Can you work these out from the model? Positions are in its coordinate system, mm. Face numbers are marked on the shaded views. A direction names the side the tool comes from. Coordinates: 2 decimals unless noted, no trailing zeros. Loops run counter-clockwise (first coordinate to the right, second up) from the corner with the lowest first, then second, coordinate; pieces in that order, holes last.
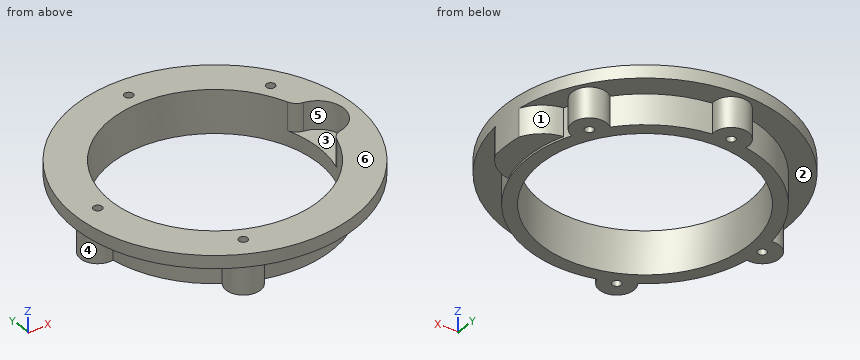
```python
from build123d import *

# Parameters (mm, degrees)
SKETCH1_R                = 32.5
SKETCH1_R_2              = 24.1
SKETCH1_R_3              = 1
RING_BODY_DEPTH          = 10
SKETCH2_R                = 6
NUB_CUT_DEPTH            = 6.5
NUB_CUT_FILLETS_3MM_R    = 3
WEIGHT_REDUCTION_DEPTH   = 7
WEIGHT_REDUCTION_2_DEPTH = 0.5


# Read off the part's stored shape, not the designer's step: Weight reduction
with BuildPart() as part:
    # Sketch1 → Ring body (new body)
    with BuildSketch(Plane.XY):
        Circle(SKETCH1_R)
        Circle(SKETCH1_R_2, mode=Mode.SUBTRACT)
        with Locations((0, 27.5)):
            Circle(SKETCH1_R_3, mode=Mode.SUBTRACT)
        with Locations((23.5226917, 14.245454545)):
            Circle(SKETCH1_R_3, mode=Mode.SUBTRACT)
        with Locations((-27.5, 0)):
            Circle(SKETCH1_R_3, mode=Mode.SUBTRACT)
        with Locations((-11.677272727, -24.897616385)):
            Circle(SKETCH1_R_3, mode=Mode.SUBTRACT)
    extrude(amount=RING_BODY_DEPTH)

    # Sketch2 → Nub cut (cut)
    with BuildSketch(Plane.XY.offset(10)):
        with Locations((24.1, 0)):
            Circle(SKETCH2_R)
    extrude(amount=-NUB_CUT_DEPTH, mode=Mode.SUBTRACT)

    # Nub cut fillets 3mm
    nub_cut_fillets_3mm_edges = [part.edges().sort_by_distance(p)[0] for p in [
        (23.353112033, 5.953331703, 6.75),
        (23.353112033, -5.953331703, 6.75),
    ]]
    fillet(nub_cut_fillets_3mm_edges, radius=NUB_CUT_FILLETS_3MM_R)

    # Weight reduction outline → Weight reduction (cut)
    with BuildSketch(Plane.XY):
        with BuildLine():
            ThreePointArc((32.28340249, -3.745920941), (29.581251517, -7.138338869), (25.606224066, -8.87306537))
            ThreePointArc((25.606224066, -8.87306537), (12.328674894, -24.13325041), (-7.817628093, -25.947922672))
            ThreePointArc((-7.817628093, -25.947922672), (-13.375785124, -28.519087859), (-14.952629097, -22.601523911))
            ThreePointArc((-14.952629097, -22.601523911), (-22.872047594, -14.535454545), (-26.812, -3.940387798))
            ThreePointArc((-26.812, -3.940387798), (-31.5, 0), (-26.812, 3.940387798))
            ThreePointArc((-26.812, 3.940387798), (-19.16259377, 19.16259377), (-3.940387798, 26.812))
            ThreePointArc((-3.940387798, 26.812), (0, 31.5), (3.940387798, 26.812))
            ThreePointArc((3.940387798, 26.812), (13.303636364, 23.60981278), (20.893010712, 17.259551077))
            ThreePointArc((20.893010712, 17.259551077), (26.944174129, 16.317520661), (24.975382732, 10.51856727))
            ThreePointArc((24.975382732, 10.51856727), (25.304182573, 9.700945537), (25.606224067, 8.87306537))
            ThreePointArc((25.606224067, 8.87306537), (29.581251517, 7.138338869), (32.28340249, 3.745920941))
            ThreePointArc((32.28340249, 3.745920941), (-32.5, 0), (32.28340249, -3.745920941))
        make_face()
    extrude(amount=WEIGHT_REDUCTION_DEPTH, mode=Mode.SUBTRACT)

    # Weight reduction 2 outline → Weight reduction 2 (cut)
    with BuildSketch(Plane.XY):
        with BuildLine():
            ThreePointArc((25.606224067, 8.87306537), (27.1, 0), (25.606224066, -8.87306537))
            ThreePointArc((25.606224066, -8.87306537), (29.581251517, -7.138338869), (32.28340249, -3.745920941))
            ThreePointArc((32.28340249, -3.745920941), (32.5, 0), (32.28340249, 3.745920941))
            ThreePointArc((32.28340249, 3.745920941), (29.581251517, 7.138338869), (25.606224067, 8.87306537))
        make_face()
    extrude(amount=WEIGHT_REDUCTION_2_DEPTH, mode=Mode.SUBTRACT)


solid = part.part
```
Item 1: On a 3-axis mill with a long thin cutter (end or side, diameter ignored), from which of +Z, -Z, +X, -X, +Y, -Y can I reach the whole of each face in a straight line? I mean the marked faces 1, 2 and 3. Say none if no direction works.
Results are:
face 1: -Z, +X
face 2: -Z
face 3: +Z
Item 2: I'm going to push flat-ended pins straight in: P1, Ø2, axis at x = 30, y = -2, coming from the -Z side; P2, Ø2, axis at x = 12.5, z = 5.5, coming from the -Y side; P3, Ø1, axis at y = -1, z = 2, coming from the +X side. Where does each tip first touch, or does it pass through?
Results are:
P1: stops at z = 0.5
P2: stops at y = -24.54
P3: stops at x = 32.5
Item 3: Suppose I cut it at C-C, the plane x = 14. Please give me the cut outline in (y, z).
Results are:
outline: (-29.33, 7) - (-23.2, 7) - (-23.2, 0) - (-19.62, 0) - (-19.62, 10) - (-29.33, 10) - close; (19.62, 0) - (23.2, 0) - (23.2, 7) - (29.33, 7) - (29.33, 10) - (19.62, 10) - close
Item 4: We'd pull the mould along Y, two halves only. Please class the marked faces 4, 5 and 6: +Y half, -Y half, draft (parallel to the pull), parting line (faces both ways), or undercut.
Results are:
face 4: parting line
face 5: undercut
face 6: draft
Item 5: Suppose I cut it at A-A, the plane y = 0. Please give me the cut outline in (x, z).
Results are:
outline: (-32.5, 7) - (-31.5, 7) - (-31.5, 0) - (-28.5, 0) - (-28.5, 10) - (-32.5, 10) - close; (-26.5, 0) - (-24.1, 0) - (-24.1, 10) - (-26.5, 10) - close; (24.1, 0) - (27.1, 0) - (27.1, 0.5) - (32.5, 0.5) - (32.5, 10) - (30.1, 10) - (30.1, 3.5) - (24.1, 3.5) - close
Item 6: I need wall thicknesses on line 1 along Y through (x, z) = (0, 3.25); line 2 along Y through (x, z) = (-27.5, 3); line 3 along Y through (x, z) = (19.5, 2.5). Which ranges of each line are inside material? Lowest first, please.
Results are:
line 1: y = -27.1 to -24.1, 24.1 to 26.5, 28.5 to 31.5
line 2: y = -4 to -1, 1 to 4
line 3: y = -18.82 to -14.16, 14.16 to 18.82
Item 7: Suppose I cut it at D-D, the plane y = -10.5. Please give me the cut outline in (x, z), plus the area to 3 significant figures.
Results are:
outline: (-30.76, 7) - (-24.98, 7) - (-24.98, 0) - (-21.69, 0) - (-21.69, 10) - (-30.76, 10) - close; (21.69, 0) - (24.98, 0) - (24.98, 7) - (30.76, 7) - (30.76, 10) - (21.69, 10) - close
area: 100 mm2
Item 8: Suppose I cut it at B-B, the plane x = 0. Please give me the cut outline in (y, z).
Results are:
outline: (-32.5, 7) - (-27.1, 7) - (-27.1, 0) - (-24.1, 0) - (-24.1, 10) - (-32.5, 10) - close; (24.1, 0) - (26.5, 0) - (26.5, 10) - (24.1, 10) - close; (28.5, 0) - (31.5, 0) - (31.5, 7) - (32.5, 7) - (32.5, 10) - (28.5, 10) - close
